Check sheet for the modelled part. Datum: model origin and axes. Units: mm. A direction names the side the tool comes from. Coordinates: 2 decimals unless noted, no trailing zeros. Loops run counter-clockwise (first coordinate to the right, second up) from the corner with the lowest first, then second, coordinate; pieces in that order, holes last. Notation, with made-up numbers: (53, 53.5) -> (100, 53.5) arc R18 cw to (100, 79.5) -> close; hole circle Ø2 at (-9.5, 1.25). An arc over 180 degrees is marked (long way). Use CSV: the item, a comma, the result in double quotes. Start each with the question number.
1. Release check for a two-part mould opening along X. For faces 1 (the face through (-23.277, -12.311, 7.93)), 2 (the face through (-10, 22, 13)), 3 (the face through (-23.17, 7.25, 1.48)) record: pulls with the +X half, pulls with the -X half, needs draft (parallel to the pull), parting line crosses it, or undercut.
2. Sectioned sample at C-C, the plane y = -9. Record the cut outline in (x, z).
3. Gauge pin test, flat ends, axial feed: pin 1 (3 mm diameter, centred on x = 4.5, z = 9.5, fed in from +Y); pin 2 (4 mm diameter, centred on x = -14, y = -0.5, fed in from +Z); pin 3 (1 mm diameter, centred on x = 3, z = 7, fed in from -Y). Record the tip position at first contact, or that the pin passes through.
4. Set-up check for faces 4 (the face through (2.731, -13.337, 7.93)), 5 (the face through (-11, 0, 0)): record each of +Z, -Z, +X, -X, +Y, -Y from which the full face is reachable in a straight line by a thin tool's end or side.
5. Thickness scan on L1, parallel to Z at x = -8, y = 0; L2, parallel to X at y = -14, z = 5; L3, parallel to Y at x = -14.5, z = 1.5. Record the ranges inside material, lowest first.
6. Sectioned sample at B-B, the plane z = 1.75. Record the cut outline in (x, y).
7. Sectioned sample at D-D, the plane z = 8.25. Record the cut outline in (x, y).
8. Sectioned sample at A-A, the plane x = 5. Record the cut outline in (y, z), and give its area (3 significant figures).
```python
from build123d import *

# Parameters (mm, degrees)
SALIENTE_EXTRUIR1_DEPTH = 3
CROQUIS2_R              = 4
SALIENTE_EXTRUIR2_DEPTH = 10


with BuildPart() as part:
    # Croquis1 → Saliente-Extruir1 (new body)
    with BuildSketch(Plane.XY):
        with BuildLine():
            Line((-27.272909543, -17.135189149), (6.546750569, -17.135189149))
            ThreePointArc((6.546750569, -17.135189149), (10.800004611, -14.76384471), (11.018886524, -9.899121172))
            Line((11.018886524, -9.899121172), (-5.890943532, 23.920538941))
            ThreePointArc((-5.890943532, 23.920538941), (-10.363079487, 26.684470963), (-14.835215442, 23.920538941))
            Line((-14.835215442, 23.920538941), (-31.745045498, -9.899121172))
            ThreePointArc((-31.745045498, -9.899121172), (-31.526163585, -14.76384471), (-27.272909543, -17.135189149))
        make_face()
    extrude(amount=SALIENTE_EXTRUIR1_DEPTH)

    # Croquis2 → Saliente-Extruir2 (add)
    with BuildSketch(Plane.XY.offset(3)):
        with Locations(Location((-10.363079487, 21.684470963, 0), (0, 0, 180))):
            Circle(CROQUIS2_R)
        with Locations(Location((-27.272909543, -12.135189149, 0), (0, 0, 180))):
            Circle(CROQUIS2_R)
        with Locations(Location((6.546750569, -12.135189149, 0), (0, 0, 180))):
            Circle(CROQUIS2_R)
    extrude(amount=SALIENTE_EXTRUIR2_DEPTH)


solid = part.part
```
Completed:
1,face 1,"undercut"
1,face 2,"needs draft"
1,face 3,"pulls with the -X half"
2,outline,"(-31.3, 0) -> (10.57, 0) -> (10.57, 3) -> (9.03, 3) -> (9.03, 13) -> (4.06, 13) -> (4.06, 3) -> (-24.79, 3) -> (-24.79, 13) -> (-29.76, 13) -> (-29.76, 3) -> (-31.3, 3) -> close"
3,pin 1,"y = -8.17"
3,pin 2,"z = 3"
3,pin 3,"y = -14.73"
4,face 4,"+Z"
4,face 5,"-Z, +X, -X, +Y, -Y"
5,L1,"0 to 3"
5,L2,"-30.81 to -23.73, 3.01 to 10.09"
5,L3,"-17.14 to 24.49"
6,outline,"(-31.75, -9.9) arc R5 ccw to (-27.27, -17.14) -> (6.55, -17.14) arc R5 ccw to (11.02, -9.9) -> (-5.89, 23.92) arc R5 ccw to (-14.84, 23.92) -> close"
7,outline,"circle Ø8 at (-27.27, -12.14); circle Ø8 at (-10.36, 21.68); circle Ø8 at (6.55, -12.14)"
8,outline,"(-17.14, 0) -> (2.14, 0) -> (2.14, 3) -> (-8.45, 3) -> (-8.45, 13) -> (-15.82, 13) -> (-15.82, 3) -> (-17.14, 3) -> close"
8,area,"132 mm²"
